Work out the finished part from the listing and answer in its coordinate system (mm). A direction names the side the tool comes from. Give positions to 0.01 mm unless a question says otherwise; leave off trailing zeros. Loops run counter-clockwise (first coordinate to the right, second up) from the corner with the lowest first, then second, coordinate; pieces in that order, holes last. Notation, with made-up numbers: (29, 71) - (60, 71) arc R27 cw to (60, 102) - close; hole circle Ø2 at (15, 58.25). An arc over 180 degrees is marked (long way). One line per question, with ' | ' between items.
from build123d import *

# Parameters (mm, degrees)
SKETCH_W        = 40
SKETCH_H        = 40
SKETCH_R        = 2.5
PAD_DEPTH       = 5
PAD001_DEPTH    = 35
SKETCH002_R     = 3
POCKET_DEPTH    = 5.001
POCKET001_DEPTH = 40.001
CHAMFER_SIZE    = 4
CHAMFER001_SIZE = 4


with BuildPart() as part:
    # Sketch → Pad (new body)
    with BuildSketch(Plane.XY):
        with Locations((20, 20)):
            Rectangle(SKETCH_W, SKETCH_H)
        with Locations((10, 30)):
            Circle(SKETCH_R, mode=Mode.SUBTRACT)
        with Locations((30, 30)):
            Circle(SKETCH_R, mode=Mode.SUBTRACT)
        with Locations((30, 10)):
            Circle(SKETCH_R, mode=Mode.SUBTRACT)
        with Locations((10, 10)):
            Circle(SKETCH_R, mode=Mode.SUBTRACT)
    extrude(amount=PAD_DEPTH)

    # Sketch001 (on Face10 of Pad) → Pad001 (join)
    with BuildSketch(Plane.XY.offset(5)):
        Polygon((0, 0), (5, 0), (5, 35), (35, 35), (35, 0), (40, 0), (40, 40), (0, 40), align=None)
    extrude(amount=PAD001_DEPTH)

    # Sketch002 (on Face17 of Pad001) → Pocket (cut, through all)
    with BuildSketch(Plane.XZ.offset(-35)):
        with Locations((20, 32.5)):
            Circle(SKETCH002_R)
        with Locations((20, 12.5)):
            Circle(SKETCH002_R)
    extrude(amount=-POCKET_DEPTH, mode=Mode.SUBTRACT)

    # Sketch003 (on Face10 of Pocket) → Pocket001 (cut, through all)
    with BuildSketch(Plane.YZ.offset(40)):
        Polygon((0, 40), (0, 5), (35, 40), align=None)
    extrude(amount=-POCKET001_DEPTH, mode=Mode.SUBTRACT)

    # Chamfer
    chamfer_edges = [part.edges().sort_by_distance(p)[0] for p in [
        (40, 37.5, 40),
        (0, 37.5, 40),
    ]]
    chamfer(chamfer_edges, length=CHAMFER_SIZE)

    # Chamfer001
    chamfer001_edges = [part.edges().sort_by_distance(p)[0] for p in [
        (40, 0, 2.5),
        (0, 0, 2.5),
    ]]
    chamfer(chamfer001_edges, length=CHAMFER001_SIZE)


solid = part.part
1. Find section A-A on x = 10. Write down the section's boundary in (y, z), then the cut area to 3 significant figures.
Evaluation:
outline: (0, 0) - (7.5, 0) - (7.5, 5) - (0, 5) - close; (12.5, 0) - (27.5, 0) - (27.5, 5) - (12.5, 5) - close; (32.5, 0) - (40, 0) - (40, 40) - (35, 40) - (35, 5) - (32.5, 5) - close | area: 325 mm2
2. Consider L1, parallel to Y at x = 10, z = 3; L2, parallel to Z at x = 20, y = 38; L3, parallel to X at y = 9.5, z = 12.5. Determine where each line is inside the solid, lowest interval first.
Evaluation:
L1: 0 to 7.5, 12.5 to 27.5, 32.5 to 40 | L2: 0 to 9.5, 15.5 to 29.5, 35.5 to 40 | L3: 0 to 5, 35 to 40
3. Find section D-D on z = 25. Write down the section's boundary in (x, y), then the cut area to 3 significant figures.
Evaluation:
outline: (0, 20) - (5, 20) - (5, 35) - (35, 35) - (35, 20) - (40, 20) - (40, 40) - (0, 40) - close | area: 350 mm2
4. Find section B-B on z = 12.5. Write down the section's boundary in (x, y), then the cut area to 3 significant figures.
Evaluation:
outline: (0, 7.5) - (5, 7.5) - (5, 35) - (17, 35) - (17, 40) - (0, 40) - close; (23, 35) - (35, 35) - (35, 7.5) - (40, 7.5) - (40, 40) - (23, 40) - close | area: 445 mm2
5. Flat-ended cylindrical pins translate along their axes: pin 1 (15 mm diameter, centred on x = 26.5, y = 20, fed in from +Z); pin 2 (9 mm diameter, centred on x = 25.5, z = 18, fed in from -Y); pin 3 (3.5 mm diameter, centred on x = 20, z = 12.5, fed in from -Y). Find the tip coordinate at first contact, or state that the pin passes through.
Evaluation:
pin 1: z = 5 | pin 2: y = 35 | pin 3: through
6. Which of the six approach directions +Z, -Z, +X, -X, +Y, -Y give full straight-line access (tool end or side, diameter ignored) to faces 5 (the flat face through (5, 25, 14)), 6 (the flat face through (40, 26, 14))?
Evaluation:
face 5: +Z, -Y | face 6: +Z, -Z, +X, +Y, -Y
7. Determine the mould class of faces 1 (the flat face through (38, 36, 38)), 2 (the flat face through (0, 26, 14)), 3 (the cylindrical face through (17.79, 37.47, 34.53)), 4 (the flat face through (20, 40, 20)) for opening direction X: +X half, -X half, draft (parallel to the pull), parting line (faces both ways), or undercut.
Evaluation:
face 1: +X half | face 2: -X half | face 3: undercut | face 4: draft
8. Find section C-C on y = 25. Write down the section's boundary in (x, z).
Evaluation:
outline: (0, 0) - (40, 0) - (40, 30) - (35, 30) - (35, 5) - (5, 5) - (5, 30) - (0, 30) - close
